```python
from build123d import *

# Parameters (mm, degrees)
BASE_FLANGE1_DEPTH      = 50.8
CUT_EXTRUDE1_DEPTH      = 76.778703488
CUT_EXTRUDE1_DEPTH_BACK = 76.778703488
SKETCH6_R               = 2.4892


# Sheet-metal steps are written as plain solids
with BuildPart() as part:
    # Sketch1 → Base-Flange1 (new body)
    with BuildSketch(Plane.XY):
        with BuildLine():
            Line((-53.2765, -6.35), (-53.2765, 5.588))
            ThreePointArc((-53.2765, 5.588), (-53.053315367, 6.126815367), (-52.5145, 6.35))
            Line((-52.5145, 6.35), (52.5145, 6.35))
            ThreePointArc((52.5145, 6.35), (53.053315367, 6.126815367), (53.2765, 5.588))
            Line((53.2765, 5.588), (53.2765, -6.35))
            Line((53.2765, -6.35), (55.5625, -6.35))
            Line((55.5625, -6.35), (55.5625, 5.588))
            ThreePointArc((55.5625, 5.588), (54.669761469, 7.743261469), (52.5145, 8.636))
            Line((52.5145, 8.636), (-52.5145, 8.636))
            ThreePointArc((-52.5145, 8.636), (-54.669761469, 7.743261469), (-55.5625, 5.588))
            Line((-55.5625, 5.588), (-55.5625, -6.35))
            Line((-55.5625, -6.35), (-53.2765, -6.35))
        make_face()
    extrude(amount=BASE_FLANGE1_DEPTH)

    # Sketch6 → Cut-Extrude1 (cut, two sides: drawn at the far end of the back side and taken through both)
    with BuildSketch(Plane(origin=(0, 0, 0), x_dir=(0, 0, -1), z_dir=(1, 0, 0)).offset(-CUT_EXTRUDE1_DEPTH_BACK)):
        with Locations((-6.35, -0.888959106)):
            Circle(SKETCH6_R)
        with Locations((-19.05, -0.888959106)):
            Circle(SKETCH6_R)
        with Locations((-31.75, -0.888959106)):
            Circle(SKETCH6_R)
        with Locations((-44.45, -0.888959106)):
            Circle(SKETCH6_R)
    extrude(amount=CUT_EXTRUDE1_DEPTH + CUT_EXTRUDE1_DEPTH_BACK, mode=Mode.SUBTRACT)


solid = part.part
```
Design review of the part built by this model. Coordinates are the model's own, in mm. A direction names the side the tool comes from. Coordinates: 2 decimals unless noted, no trailing zeros. Order: outer loops, then holes, each group sorted by start corner. A loop starts at its lowest first (then second) coordinate and runs counter-clockwise, first axis right, second up. Notation, with made-up numbers: (-9, -39.5) - (5, -39.5) arc R15 cw to (5, -30.5) - close; hole circle Ø9 at (57, 70.25). An arc over 180 degrees is marked (long way). Answer in a Markdown table with one row per item.
(1) Wall thickness on line 1 along X through (y, z) = (0.75, 16); line 2 along Y through (x, z) = (54.85, 44.45); line 3 along Y through (x, z) = (53.85, 44.45): over which ranges is each line inside the solid? List them lowest first. Write a range as from..to.
Checked values:
| item | result |
|---|---|
| line 1 | -55.56..-53.28, 53.28..55.56 |
| line 2 | -6.35..-3.38, 1.6..7.55 |
| line 3 | -6.35..-3.38, 1.6..8.33 |
(2) Consider section A-A on z = 6.35. State the section outline as (x, y) points, plus the area to 3 significant figures.
Checked values:
| item | result |
|---|---|
| outline | (-55.56, -6.35) - (-53.28, -6.35) - (-53.28, -3.38) - (-55.56, -3.38) - close; (-55.56, 1.6) - (-53.28, 1.6) - (-53.28, 5.59) arc R0.76 cw to (-52.51, 6.35) - (52.51, 6.35) arc R0.76 cw to (53.28, 5.59) - (53.28, 1.6) - (55.56, 1.6) - (55.56, 5.59) arc R3.05 ccw to (52.51, 8.64) - (-52.51, 8.64) arc R3.05 ccw to (-55.56, 5.59) - close; (53.28, -6.35) - (55.56, -6.35) - (55.56, -3.38) - (53.28, -3.38) - close |
| area | 286 mm^2 |
(3) Consider section B-B on x = -29. State the section outline as (y, z) points, plus the area to 3 significant figures.
Checked values:
| item | result |
|---|---|
| outline | (6.35, 0) - (8.64, 0) - (8.64, 50.8) - (6.35, 50.8) - close |
| area | 116 mm^2 |
(4) Clearance check with flat-ended pins moving along their axes: pin 1 (4.5 mm diameter, centred on y = -0.89, z = 31.75, fed in from -X); pin 2 (1.5 mm diameter, centred on x = 8.5, z = 33, fed in from -Y). State where each tip first meets the part, or that it passes through.
Checked values:
| item | result |
|---|---|
| pin 1 | through |
| pin 2 | y = 6.35 |
(5) For faces 4 (the cylindrical face through (-54.436, -0.141, 3.976)), 5 (the flat face through (-53.276, 0, 25)), list the 3-axis set-ups (+Z, -Z, +X, -X, +Y, -Y) from which the entire face can be reached by the end or side of a thin tool; tool diameter is ignored.
Checked values:
| item | result |
|---|---|
| face 4 | +X, -X |
| face 5 | +Z, -Z, -Y |
(6) The part is to be moulded in two halves that separate along Z. For faces 1 (the cylindrical face through (54.403, -0.78, 34.237)), 2 (the flat face through (54, -6.35, 25)), 3 (the flat face through (-8, 7, 0)), say which applies: released by +Z, released by -Z, zero draft, split by the parting line, or undercut.
Checked values:
| item | result |
|---|---|
| face 1 | undercut |
| face 2 | zero draft |
| face 3 | released by -Z |
(7) Consider section C-C on z = 33. State the section outline as (x, y) points.
Checked values:
| item | result |
|---|---|
| outline | (-55.56, -6.35) - (-53.28, -6.35) - (-53.28, -3.04) - (-55.56, -3.04) - close; (-55.56, 1.26) - (-53.28, 1.26) - (-53.28, 5.59) arc R0.76 cw to (-52.51, 6.35) - (52.51, 6.35) arc R0.76 cw to (53.28, 5.59) - (53.28, 1.26) - (55.56, 1.26) - (55.56, 5.59) arc R3.05 ccw to (52.51, 8.64) - (-52.51, 8.64) arc R3.05 ccw to (-55.56, 5.59) - close; (53.28, -6.35) - (55.56, -6.35) - (55.56, -3.04) - (53.28, -3.04) - close |
